from build123d import *

# Parameters (mm, degrees)
BOSS_EXTRUDE1_DEPTH = 3.85
CHAMFER1_SIZE       = 1


with BuildPart() as part:
    # Sketch1 → Boss-Extrude1 (new body)
    with BuildSketch(Plane(origin=(0, 0, 0), x_dir=(1, 0, 0), z_dir=(0, 1, 0))):
        Polygon((17.46076087, -11.925), (11.925, -17.46076087), (1.925, -17.46076087), (1.925, -12.46076087), (-1.925, -12.46076087), (-1.925, -17.46076087), (-11.925, -17.46076087), (-17.46076087, -11.925), (-17.46076087, -1.925), (-12.46076087, -1.925), (-12.46076087, 1.925), (-17.46076087, 1.925), (-17.46076087, 11.925), (-11.925, 17.46076087), (-1.925, 17.46076087), (-1.925, 12.46076087), (1.925, 12.46076087), (1.925, 17.46076087), (11.925, 17.46076087), (17.46076087, 11.925), (17.46076087, 1.925), (12.46076087, 1.925), (12.46076087, -1.925), (17.46076087, -1.925), align=None)
    extrude(amount=BOSS_EXTRUDE1_DEPTH)

    # Chamfer1
    chamfer1_edges = [part.edges().sort_by_distance(p)[0] for p in [
        (17.46076087, 1.925, -1.925),
        (17.46076087, 1.925, 1.925),
        (1.925, 1.925, 17.46076087),
        (-1.925, 1.925, 17.46076087),
        (-17.46076087, 1.925, 1.925),
        (-17.46076087, 1.925, -1.925),
        (-1.925, 1.925, -17.46076087),
        (1.925, 1.925, -17.46076087),
    ]]
    chamfer(chamfer1_edges, length=CHAMFER1_SIZE)


solid = part.part
Input: part model. Units: mm. Frame: model coordinates. A direction names the side the tool comes from. Give positions to 0.01 mm unless a question says otherwise; leave off trailing zeros. Write each loop counter-clockwise with the first axis right and the second up, starting at its lowest first coordinate (ties: lowest second). Pieces come first, ordered by that corner, then holes. Notation, with made-up numbers: M 4.25,51.25 L 14.25,51.25 A15 ccw 14.25,55.25 Z; hole C 3,77 d6. An arc over 180 degrees is marked long. Use one line per item in the form item = value.
1. Cut plane D-D on x = 1. Return loops of the section in (y, z), and give its area (3 significant figures).
Outcome:
outline = M 0,-12.46 L 3.85,-12.46 L 3.85,12.46 L 0,12.46 Z
area = 95.9 mm²
2. Reachability of faces 1 (the face through (1.925, 2, -14)), 2 (the face through (2.418, 1.898, 16.954)), 3 (the face through (7, 2, 17.461)), 4 (the face through (14, 2, 1.925)), 5 (the face through (-14, 2, -1.925)) from +Z, -Z, +X, -X, +Y, -Y: full face, straight path, thin tool, end or side. Return the list, or none.
Outcome:
face_1 = -Z, +Y, -Y
face_2 = +Z, +Y, -Y
face_3 = +Z, +X, -X, +Y, -Y
face_4 = +X, +Y, -Y
face_5 = -X, +Y, -Y
3. Ray query, L1, parallel to Z at x = 0, y = 0.95; L2, parallel to X at y = 0.2, z = 13 (3 decimals); L3, parallel to X at y = 1.8, z = -12.5 (3 decimals). Return the intervals inside material, ascending.
Outcome:
L1 = -12.46 to 12.46
L2 = -16.386 to -1.925, 1.925 to 16.386
L3 = -16.886 to -1.925, 1.925 to 16.886
4. Cut plane A-A on x = 13. Return loops of the section in (y, z) (3 decimals), and give its area (3 significant figures).
Outcome:
outline = M 0,-16.386 L 3.85,-16.386 L 3.85,-1.925 L 0,-1.925 Z; M 0,1.925 L 3.85,1.925 L 3.85,16.386 L 0,16.386 Z
area = 111 mm²
5. Cut plane C-C on z = -15. Return loops of the section in (x, y) (3 decimals), and give its area (3 significant figures).
Outcome:
outline = M -14.386,0 L -1.925,0 L -1.925,3.85 L -14.386,3.85 Z; M 1.925,0 L 14.386,0 L 14.386,3.85 L 1.925,3.85 Z
area = 95.9 mm²
6. First-contact query: P1, Ø1.9, axis at y = 1.5, z = -15.5, coming from the +X side; P2, Ø1.9, axis at x = -14.5, y = 2, coming from the +Z side; P3, Ø1.9, axis at x = -15, y = 2, coming from the -Z side; P4, Ø3, axis at x = -3, z = -0.5, coming from the -Y side. Flat tips, straight axial feed; report the tip coordinate or a pass-through.
Outcome:
P1 = 14.84
P2 = 15.84
P3 = -15.34
P4 = 0
7. Mould query, pull axis X, two halves, no side actions, for faces 6 (the face through (17.461, 2, -7)), 7 (the face through (2.432, 1.898, -16.968)), 8 (the face through (-17.461, 2, 7)), 9 (the face through (-14, 2, 1.925)). Classes: released by +X, released by -X, zero draft, split by the parting line, or undercut.
Outcome:
face_6 = released by +X
face_7 = undercut
face_8 = released by -X
face_9 = zero draft
